from build123d import *

# Parameters (mm, degrees)
SKETCH1_R           = 12.25
BOSS_EXTRUDE1_DEPTH = 11
SKETCH2_R           = 16
BOSS_EXTRUDE2_DEPTH = 2
SKETCH4_R           = 10
BOSS_EXTRUDE4_DEPTH = 1
SKETCH5_R           = 8.5
BOSS_EXTRUDE5_DEPTH = 12
SKETCH6_R           = 3
CUT_EXTRUDE1_DEPTH  = 100
CHAMFER1_SIZE       = 1
BOSS_EXTRUDE6_START = 2
SKETCH3_R           = 16
BOSS_EXTRUDE6_DEPTH = 2
CUT_EXTRUDE2_START  = -10
SKETCH7_R           = 3
CUT_EXTRUDE2_DEPTH  = 10


with BuildPart() as part:
    # Sketch1 → Boss-Extrude1 (new body)
    with BuildSketch(Plane.XY):
        Circle(SKETCH1_R)
    extrude(amount=BOSS_EXTRUDE1_DEPTH)

    # Sketch2 → Boss-Extrude2 (add)
    with BuildSketch(Plane(origin=(0, 0, 0), x_dir=(-1, 0, 0), z_dir=(0, 0, -1))):
        Circle(SKETCH2_R)
    extrude(amount=BOSS_EXTRUDE2_DEPTH)

    # Sketch4 → Boss-Extrude4 (add)
    with BuildSketch(Plane(origin=(0, 0, -2), x_dir=(-1, 0, 0), z_dir=(0, 0, -1))):
        Circle(SKETCH4_R)
    extrude(amount=BOSS_EXTRUDE4_DEPTH)

    # Sketch5 → Boss-Extrude5 (add)
    with BuildSketch(Plane(origin=(0, 0, -3), x_dir=(-1, 0, 0), z_dir=(0, 0, -1))):
        Circle(SKETCH5_R)
    extrude(amount=BOSS_EXTRUDE5_DEPTH)

    # Sketch6 → Cut-Extrude1 (cut)
    with BuildSketch(Plane(origin=(0, 0, -15), x_dir=(-1, 0, 0), z_dir=(0, 0, -1))):
        Circle(SKETCH6_R)
    extrude(amount=-CUT_EXTRUDE1_DEPTH, mode=Mode.SUBTRACT)

    # Chamfer1
    chamfer1_edges = [part.edges().sort_by_distance(p)[0] for p in [
        (3, 0, -15),
    ]]
    chamfer(chamfer1_edges, length=CHAMFER1_SIZE)

    # Sketch3 → Boss-Extrude6 (add)
    with BuildSketch(Plane.XY.offset(11).offset(BOSS_EXTRUDE6_START)):
        with Locations(Location((0, 0, 0), (0, 0, 180))):
            Circle(SKETCH3_R)
    extrude(amount=-BOSS_EXTRUDE6_DEPTH)

    # Sketch7 → Cut-Extrude2 (cut)
    with BuildSketch(Plane.XY.offset(13).offset(CUT_EXTRUDE2_START)):
        with Locations(Location((0, 0, 0), (0, 0, 180))):
            Circle(SKETCH7_R)
    extrude(amount=CUT_EXTRUDE2_DEPTH, mode=Mode.SUBTRACT)


solid = part.part
Model file for the job. Use its own axes, mm. A direction names the side the tool comes from. Give positions to 0.01 mm unless a question says otherwise; leave off trailing zeros. Order: outer loops, then holes, each group sorted by start corner. A loop starts at its lowest first (then second) coordinate and runs counter-clockwise, first axis right, second up. Notation, with made-up numbers: (70, -2.5) - (110, -2.5) arc R22 ccw to (110, 24.5) - close; hole circle Ø9 at (14, 85). An arc over 180 degrees is marked (long way). One line per item, written item: value.
Item 1: Slice it at C-C (z = -7.5). List the corners of the cut face in (x, y).
Response values:
outline: circle Ø17 at (0, 0); hole circle Ø6 at (0, 0)
Item 2: Two-plate mould, pull along Z, no slides. Class faces 4 (the cylindrical face through (6.586, 10.329, 5.423)), 5 (the cylindrical face through (-4.57, 7.167, -8.916)), 6 (the flat face through (4.5, -7.4, -3)), 7 (the flat face through (4, 12, 11)): released by +Z, released by -Z, zero draft, split by the parting line, or undercut.
Response values:
face 4: undercut
face 5: zero draft
face 6: released by -Z
face 7: undercut
Item 3: Slice it at A-A (x = 0). List the corners of the cut face in (y, z), then the cut area to 4 significant figures.
Response values:
outline: (-16, -2) - (-10, -2) - (-10, -3) - (-8.5, -3) - (-8.5, -15) - (-4, -15) - (-3, -14) - (-3, 13) - (-16, 13) - (-16, 11) - (-12.25, 11) - (-12.25, 0) - (-16, 0) - close; (3, -14) - (4, -15) - (8.5, -15) - (8.5, -3) - (10, -3) - (10, -2) - (16, -2) - (16, 0) - (12.25, 0) - (12.25, 11) - (16, 11) - (16, 13) - (3, 13) - close
area: 452.5 mm2
Item 4: Wall check: line 1 (Z direction, x = -15, y = 3); line 2 (Y direction, x = 0, z = 3); line 3 (Y direction, x = 0, z = -1). Give the ranges that are in metal, low to high.
Response values:
line 1: -2 to 0, 11 to 13
line 2: -12.25 to -3, 3 to 12.25
line 3: -16 to -3, 3 to 16
Item 5: Pin check, flat tips, straight feed: pin 1 Ø2 at (x, z) = (1, -11) entering from +Y; pin 2 Ø3 at (x, y) = (10.5, 12) entering from -Z; pin 3 Ø1 at (x, z) = (-10.5, -10.5) entering from +Y; pin 4 Ø7 at (x, y) = (0, 0) entering from -Z. Stop position of each tip, or through.
Response values:
pin 1: y = 8.5
pin 2: z = -2
pin 3: through
pin 4: z = -14.5
Item 6: Tool access for faces 1 (the flat face through (4, -12, 0)), 2 (the flat face through (-10.4, 0.2, -2)), 3 (the cylindrical face through (3.47, 15.62, 12.01)): list every direction of +Z, -Z, +X, -X, +Y, -Y with a clear straight run to the whole face (end or side of a thin tool).
Response values:
face 1: none
face 2: -Z
face 3: +Z, -Z
Item 7: Slice it at D-D (y = 10.5). List the corners of the cut face in (x, z).
Response values:
outline: (-12.07, -2) - (12.07, -2) - (12.07, 0) - (6.31, 0) - (6.31, 11) - (12.07, 11) - (12.07, 13) - (-12.07, 13) - (-12.07, 11) - (-6.31, 11) - (-6.31, 0) - (-12.07, 0) - close
